Input: dimensioned drawing with shaded views. Units: mm. Origin: part minimum x, y, z. A direction names the side the tool comes from. Give positions to 0.01 mm unless a question says otherwise; leave off trailing zeros. Write each loop counter-clockwise with the first axis right and the second up, starting at its lowest first coordinate (ties: lowest second). Pieces come first, ordered by that corner, then holes. Notation, with made-up numbers: M 60.5,27.25 L 104.5,27.25 A32 cw 104.5,65.25 Z; hole C 57,66.5 d4. An arc over 180 degrees is marked long. Answer as a JSON object with one key per item and string values.
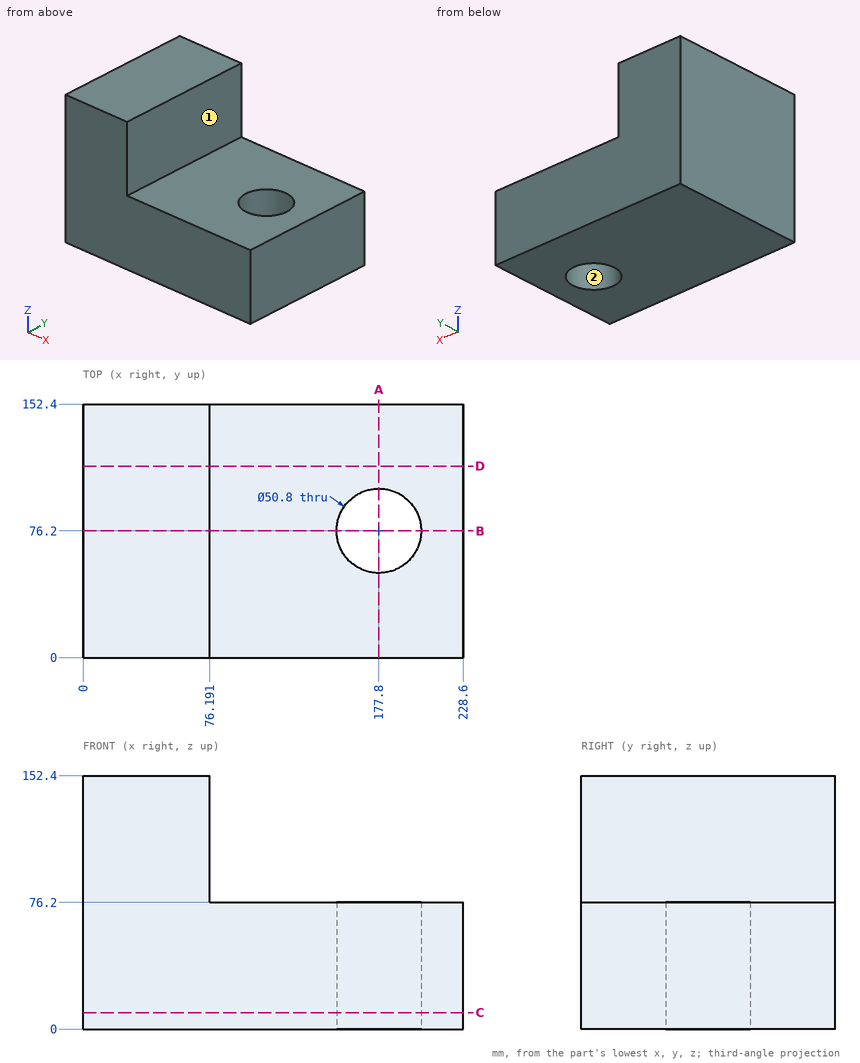
1) Cut plane D-D on y = 115. Return loops of the section in (x, z).
Geometry check:
{"outline": "M 0,0 L 228.6,0 L 228.6,76.2 L 76.19,76.2 L 76.19,152.4 L 0,152.4 Z"}
2) Cut plane A-A on x = 177.8. Return loops of the section in (y, z).
Geometry check:
{"outline": "M 0,0 L 50.8,0 L 50.8,76.2 L 0,76.2 Z; M 101.6,0 L 152.4,0 L 152.4,76.2 L 101.6,76.2 Z"}
3) Set-up query: the marked faces 1 and 2. Return all of +Z, -Z, +X, -X, +Y, -Y with unobstructed straight access to the full face (end or side cutting, diameter ignored); none if empty.
Geometry check:
{"face 1": "+Z, +X, +Y, -Y", "face 2": "+Z, -Z"}
4) Line query: line 1 (X direction, y = 76.5, z = 51.5); line 2 (Y direction, x = 177, z = 51); line 3 (X direction, y = 18, z = 131). Output: solid intervals per line, ascending. Write a range as from..to.
Geometry check:
{"line 1": "x = 0..152.4, 203.2..228.6", "line 2": "y = 0..50.81, 101.59..152.4", "line 3": "x = 0..76.19"}
5) Contact query for a flat-ended pin moving along its axis: P1, Ø10, axis at x = 84, y = 41, coming from the +Z side. Output: stop coordinate, or through.
Geometry check:
{"P1": "stops at z = 76.2"}
6) Cut plane C-C on z = 10. Return loops of the section in (x, y).
Geometry check:
{"outline": "M 0,0 L 228.6,0 L 228.6,152.4 L 0,152.4 Z; hole C 177.8,76.2 d50.8"}
7) Cut plane B-B on y = 76.2. Return loops of the section in (x, z), and give its area (3 significant figures).
Geometry check:
{"outline": "M 0,0 L 152.4,0 L 152.4,76.2 L 76.19,76.2 L 76.19,152.4 L 0,152.4 Z; M 203.2,0 L 228.6,0 L 228.6,76.2 L 203.2,76.2 Z", "area": "19,400 mm2"}
